Input: part model. Units: mm. Frame: model coordinates. A direction names the side the tool comes from. Round coordinates to 2 decimals unless told otherwise and drop trailing zeros. Loops run counter-clockwise (first coordinate to the right, second up) from the corner with the lowest first, then second, coordinate; pieces in that order, holes last. Notation, with made-up numbers: M 40,-19 L 99,-19 A21 ccw 99,17 Z; hole C -9.75,3 d8. An arc over 180 degrees is marked long. Return JSON: item names as keys, results as strings. Group by question number.
1) Access query for faces 1 (the face through (108.26, 21.83, 0.45)), 2 (the face through (79, 42, 1.905)). Directions: +Z, -Z, +X, -X, +Y, -Y. A direction counts if a zero-diameter tool reaches every point of the face in a straight line with its end or side. Return the directions, or none.
2) Section A-A (y = 28). Output: boundary loops of the cut face in (x, z) (3 decimals).
3) Material intervals for line 1 (X direction, y = 52.5, z = 2.6); line 2 (Y direction, x = 46.99, z = 0.5); line 3 (X direction, y = 20, z = 0.85), sorted ascending. Write a range as from..to.
4) Contact query for flat-ended pins moving along their axis: P1, Ø8, axis at x = 72, y = 15, coming from the -Z side; P2, Ø5, axis at x = 78.74, y = 21.54, coming from the +Z side. Output: stop coordinate, or through.
5) Section B-B (x = 110.49). Count the separate pieces of the cut face and the enclosed holes in it, plus the area to 3 significant figures.
6) Mould query, pull axis Y, two halves, no side actions, for faces 3 (the face through (61, 0, 2)), 4 (the face through (79, 66, 1.905)), 5 (the face through (108.971, 61.728, 0.939)). Classes: +Y half, -Y half, draft (parallel to the pull), parting line (faces both ways), or undercut.
Autodesk Inventor part; units mm, degrees
ref_plane "YZ Plane" through (0, 0, 0) normal (1, 0, 0) x (0, 1, 0)
ref_plane "XZ Plane" through (0, 0, 0) normal (0, 1, 0) x (-1, 0, 0)
ref_plane "XY Plane" through (0, 0, 0) normal (0, 0, 1) x (1, 0, 0)
sketch "Sketch1" plane through (0, 0, 0) normal (0, 0, 1) x (1, 0, 0)
  line L0 (0, 0) -> (123.19, 0)
  line L1 (123.19, 0) -> (123.19, 69.85)
  line L2 (123.19, 69.85) -> (0, 69.85)
  line L3 (0, 69.85) -> (0, 0)
  dimension "d0" = 69.85
  dimension "d1" = 123.19
extrude "Extrusion1" add sketch "Sketch1" along normal blind 3.175
sketch "Sketch2" plane through (0, 0, 3.175) normal (0, 0, 1) x (1, 0, 0)
  line L0 (123.19, 69.85) -> (0, 69.85)
  line L1 (0, 69.85) -> (0, 0)
  point P0 (15.24, 60.071)
  point P1 (46.99, 60.071)
  point P2 (78.74, 60.071)
  point P3 (110.49, 60.071)
  dimension "d5" = 9.779
  dimension "d6" = 15.24
  dimension "d7" = 31.75
  dimension "d8" = 31.75
  dimension "d9" = 31.75
hole "Hole1" at (15.24, 60.071, 3.175) at (46.99, 60.071, 3.175) at (78.74, 60.071, 3.175) at (110.49, 60.071, 3.175) direction (0, 0, -1) diameter 4.4958 end through all
sketch "Sketch3" plane through (0, 0, 3.175) normal (0, 0, 1) x (1, 0, 0)
  circle A0 centre (110.49, 60.071) radius 2.2479
  circle A1 centre (46.99, 60.071) radius 2.2479
  circle A2 centre (15.24, 60.071) radius 2.2479
  circle A3 centre (78.74, 60.071) radius 2.2479
  line L0 (0, 0) -> (123.19, 0)
  line L1 (123.19, 0) -> (123.19, 69.85)
  line L2 (123.19, 69.85) -> (0, 69.85)
  line L3 (0, 69.85) -> (0, 0)
  point P0 (15.24, 21.5392)
  point P1 (46.99, 21.5392)
  point P2 (78.74, 21.5392)
  point P3 (110.49, 21.5392)
hole "Hole2" at (15.24, 21.5392, 3.175) at (46.99, 21.5392, 3.175) at (78.74, 21.5392, 3.175) at (110.49, 21.5392, 3.175) direction (0, 0, -1) diameter 4.4958 end through all countersink diameter 8.4328 countersink angle 82
sketch "Sketch4" plane through (0, 0, 0) normal (0, 0, -1) x (-1, 0, 0)
  circle A0 centre (-78.74, 21.5392) radius 2.2479
  circle A1 centre (-15.24, 21.5392) radius 2.2479
  circle A2 centre (-46.99, 21.5392) radius 2.2479
  circle A3 centre (-110.49, 21.5392) radius 2.2479
  circle A4 centre (-78.74, 60.071) radius 2.2479
  circle A5 centre (-15.24, 60.071) radius 2.2479
  circle A6 centre (-46.99, 60.071) radius 2.2479
  circle A7 centre (-110.49, 60.071) radius 2.2479
  line L0 (0, 0) -> (-123.19, 0)
  line L1 (0, 69.85) -> (0, 0)
  line L2 (-123.19, 69.85) -> (0, 69.85)
  line L3 (-123.19, 0) -> (-123.19, 69.85)
  point P0 (-110.49, 9.271)
  point P1 (-78.74, 9.271)
  point P2 (-46.99, 9.271)
  point P3 (-15.24, 9.271)
  dimension "d26" = 50.8
hole "Hole3" at (110.49, 9.271, 0) at (78.74, 9.271, 0) at (46.99, 9.271, 0) at (15.24, 9.271, 0) direction (0, 0, 1) diameter 4.4958 end through all countersink diameter 8.4328 countersink angle 82
sketch "Sketch5" plane through (0, 0, 3.175) normal (0, 0, 1) x (1, 0, 0)
  circle A0 centre (46.99, 9.271) radius 2.2479 construction
  circle A1 centre (110.49, 9.271) radius 2.2479 construction
  circle A2 centre (78.74, 9.271) radius 2.2479 construction
  circle A3 centre (15.24, 9.271) radius 2.2479 construction
  circle A4 centre (78.74, 21.5392) radius 4.2164 construction
  circle A5 centre (15.24, 21.5392) radius 4.2164 construction
  circle A6 centre (46.99, 21.5392) radius 4.2164 construction
  circle A7 centre (110.49, 21.5392) radius 4.2164 construction
  circle A8 centre (78.74, 60.071) radius 2.2479 construction
  circle A9 centre (15.24, 60.071) radius 2.2479 construction
  circle A10 centre (46.99, 60.071) radius 2.2479 construction
  circle A11 centre (110.49, 60.071) radius 2.2479 construction
  line L0 (0, 0) -> (123.19, 0) construction
  line L1 (123.19, 0) -> (123.19, 69.85) construction
  line L2 (123.19, 69.85) -> (0, 69.85) construction
  line L3 (0, 69.85) -> (0, 0) construction
  circle A12 centre (15.24, 21.5392) radius 2.2479
  line L4 (12.9921, 69.85) -> (12.9921, 0)
  line L5 (17.4879, 69.85) -> (17.4879, 0)
  line L6 (12.9921, 69.85) -> (17.4879, 69.85)
  line L7 (12.9921, 0) -> (17.4879, 0)
  line L8 (0, 0) -> (123.19, 0)
  circle A13 centre (15.24, 60.071) radius 2.2479
extrude "Extrusion2" cut sketch "Sketch5" against normal blind 1.27 contours L5 L7 L4 A12 | A12 L4 A13 L5 | A13 L4 L6 L5
pattern_linear "Rectangular Pattern1" count 4 spacing 31.75 along (1, 0, 0) of "Extrusion2"
properties part number "talon stack zip tie mount" material "ABS Plastic"
Returned:
{
 "1": {"face 1": "+Z, -Z", "face 2": "+Z, +Y, -Y"},
 "2": {"outline": "M 0,0 L 123.19,0 L 123.19,3.175 L 112.738,3.175 L 112.738,1.905 L 108.242,1.905 L 108.242,3.175 L 80.988,3.175 L 80.988,1.905 L 76.492,1.905 L 76.492,3.175 L 49.238,3.175 L 49.238,1.905 L 44.742,1.905 L 44.742,3.175 L 17.488,3.175 L 17.488,1.905 L 12.992,1.905 L 12.992,3.175 L 0,3.175 Z"},
 "3": {"line 1": "x = 0..12.99, 17.49..44.74, 49.24..76.49, 80.99..108.24, 112.74..123.19", "line 2": "y = 0..5.49, 13.05..19.29, 23.79..57.82, 62.32..69.85", "line 3": "x = 0..13.6, 16.88..45.35, 48.63..77.1, 80.38..108.85, 112.13..123.19"},
 "4": {"P1": "stops at z = 0", "P2": "stops at z = 1.2"},
 "5": {"separate pieces": "4", "enclosed holes": "0", "area": "102 mm^2"},
 "6": {"face 3": "-Y half", "face 4": "draft", "face 5": "undercut"}
}
